```python
from build123d import *

# Parameters (mm, degrees)
SKETCH_R     = 7.5
PAD_DEPTH    = 1
SKETCH001_R  = 6.5
PAD001_DEPTH = 4
SKETCH002_R  = 2
POCKET_DEPTH = 5.001
FILLET_R     = 0.1


with BuildPart() as part:
    # Sketch → Pad (new body)
    with BuildSketch(Plane.XY):
        Circle(SKETCH_R)
    extrude(amount=PAD_DEPTH)

    # Sketch001 → Pad001 (new body)
    with BuildSketch(Plane.XY.offset(1)):
        with Locations((0.018028, -0.002987)):
            Circle(SKETCH001_R)
    extrude(amount=PAD001_DEPTH)

    # Sketch002 → Pocket (cut, through all)
    with BuildSketch(Plane.XY.offset(5)):
        Circle(SKETCH002_R)
    extrude(amount=-POCKET_DEPTH, mode=Mode.SUBTRACT)

    # Fillet
    fillet_edges = [part.edges().sort_by_distance(p)[0] for p in [
        (-7.5, 0, 1),
        (-7.5, 0, 0),
        (-6.481972, -0.002987, 5),
    ]]
    fillet(fillet_edges, radius=FILLET_R)


solid = part.part
```
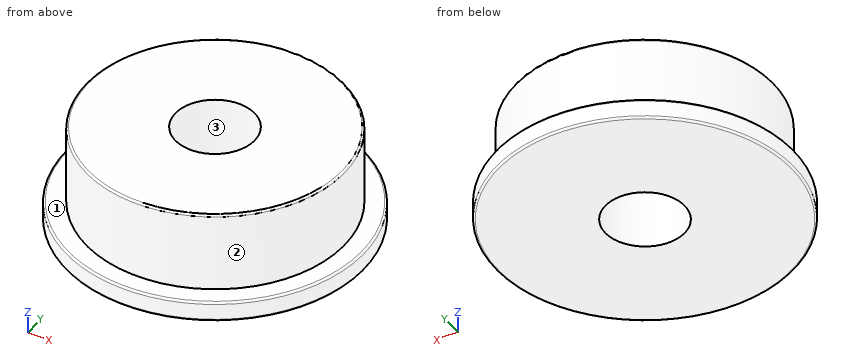
Work out the finished part from the listing and answer in its coordinate system (mm). Face numbers are marked on the shaded views. Round coordinates to 2 decimals unless told otherwise and drop trailing zeros. Write each loop counter-clockwise with the first axis right and the second up, starting at its lowest first coordinate (ties: lowest second). Pieces come first, ordered by that corner, then holes. Notation, with made-up numbers: (33.5, 85.25) -> (76.5, 85.25) arc R18 cw to (76.5, 100.25) -> close; hole circle Ø2 at (81.5, 41). An arc over 180 degrees is marked (long way). Write each question's results on one line, items separated by ' | '.
Q1. Section A-A, the plane z = 0.55 is taken. Write down the section's boundary in (x, y), then the cut area to 3 significant figures.
Data:
outline: circle Ø15 at (0, 0); hole circle Ø4 at (0, 0) | area: 164 mm^2
Q2. Flat-ended cylindrical pins translate along their axes: P1, Ø3, axis at x = 0, y = 0, coming from the +Z side; P2, Ø3, axis at y = -5, z = 3.5, coming from the +X side; P3, Ø3, axis at x = -3, z = 1.5, coming from the -Y side. Find the tip coordinate at first contact, or state that the pin passes through.
Data:
P1: through | P2: x = 5.5 | P3: y = -7.32
Q3. Determine the mould class of the marked faces 1, 2 and 3 for opening direction Y: released by +Y, released by -Y, zero draft, split by the parting line, or undercut.
Data:
face 1: zero draft | face 2: split by the parting line | face 3: undercut
Q4. Section B-B, the plane z = 2.6 is taken. Write down the section's boundary in (x, y), then the cut area to 3 significant figures.
Data:
outline: circle Ø13 at (0.02, 0); hole circle Ø4 at (0, 0) | area: 120 mm^2
Q5. Straight lines are drawn through the part: line 1 along Y through (x, z) = (0, 1.75); line 2 along Y through (x, z) = (-1, 3.6); line 3 along X through (y, z) = (-1.25, 4.7). For each, find the intervals that lie inside material, in ascending order. Write a range as [from, to].
Data:
line 1: [-6.5, -2], [2, 6.5] | line 2: [-6.42, -1.73], [1.73, 6.42] | line 3: [-6.36, -1.56], [1.56, 6.4]
